Check sheet for the drawn part. Datum: minimum x, y, z corner. Units: mm. A direction names the side the tool comes from. Give positions to 0.01 mm unless a question says otherwise; leave off trailing zeros. Write each loop counter-clockwise with the first axis right and the second up, starting at its lowest first coordinate (ties: lowest second). Pieces come first, ordered by that corner, then holes.
(1) Thickness scan on line 1 along Z through (x, y) = (4, 1.35); line 2 along X through (y, z) = (5.5, 8.25); line 3 along X through (y, z) = (0.5, 4.5) (1 decimal). Record the ranges inside material, lowest first.
(2) Cross-section at D-D (z = 4). Record the boundary of the cut face in (x, y).
(3) Cross-section at B-B (y = 6.5). Record the boundary of the cut face in (x, z).
(4) Tool access check on the marked faces 5, 6 and 7. Record the directions out of +Z, -Z, +X, -X, +Y, -Y that give a thin tool (end or side, any length) a straight path to the whole face; none if there is none.
(5) Cross-section at C-C (y = 1.75). Record the boundary of the cut face in (x, z).
(6) Mould release check, pull along X, two halves, no side actions. Record for the marked faces 1, 2, 3 and 4: +X half, -X half, draft (parallel to the pull), parting line (faces both ways), or undercut.
(7) Depth check by flat-ended pin: P1, Ø1, axis at y = 6.5, z = 4.5, coming from the +X side; P2, Ø2.5, axis at x = 4, z = 4, coming from the -Y side; P3, Ø1.2, axis at x = 9, y = 5, coming from the -Z side; P4, Ø1.2, axis at x = 3, y = 1, coming from the +Z side. Enter the tip coordinate at first touch or a pass-through.
(8) Cross-section at A-A (x = 4). Record the boundary of the cut face in (y, z).
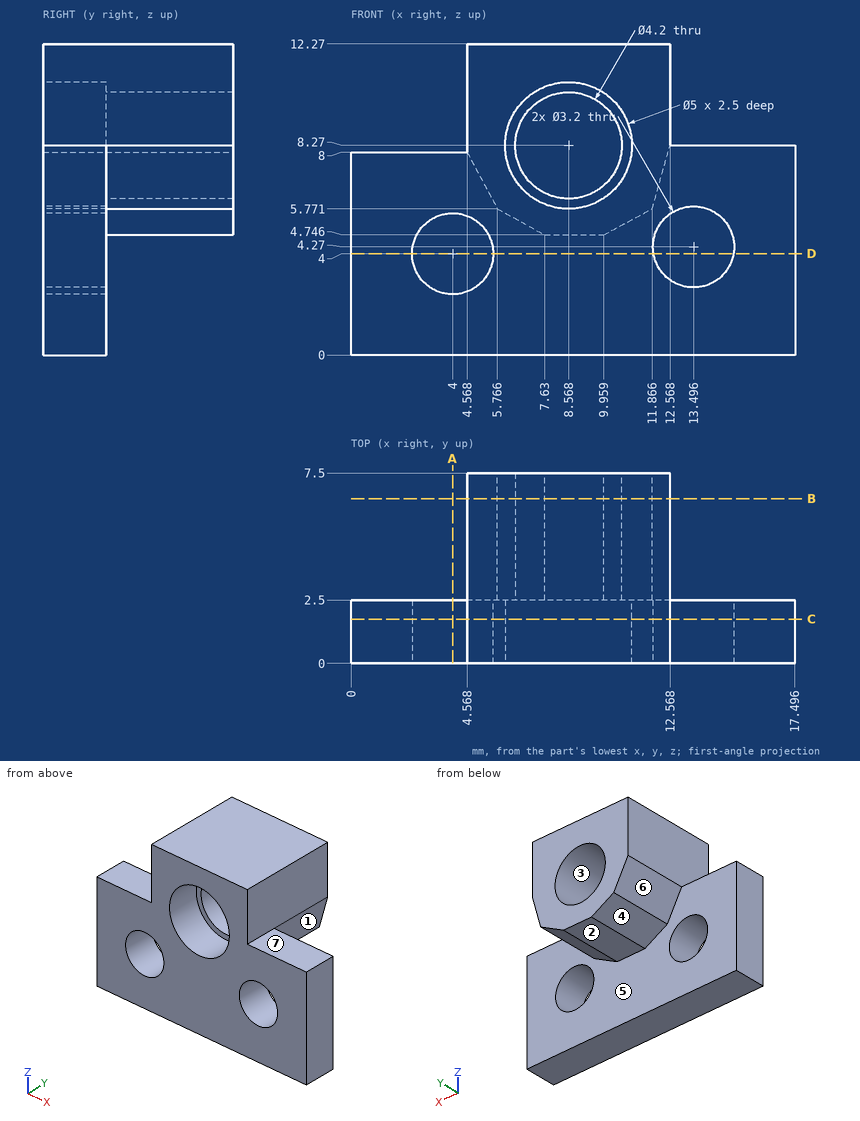
Reply:
1. line 1: z = 0 to 2.4, 5.6 to 8
1. line 2: x = 4.57 to 6.47, 10.67 to 12.56
1. line 3: x = 0 to 2.5, 5.5 to 11.9, 15.1 to 17.5
2. outline: (0, 0) - (2.4, 0) - (2.4, 2.5) - (0, 2.5) - close; (5.6, 0) - (11.92, 0) - (11.92, 2.5) - (5.6, 2.5) - close; (15.07, 0) - (17.5, 0) - (17.5, 2.5) - (15.07, 2.5) - close
3. outline: (4.57, 8) - (5.77, 5.77) - (7.63, 4.75) - (9.96, 4.75) - (11.87, 5.77) - (12.57, 8.27) - (12.57, 12.27) - (4.57, 12.27) - close; hole circle Ø4.2 at (8.57, 8.27)
4. face 5: -Z, +Y
4. face 6: -Z, -X, +Y
4. face 7: +Z, +X, +Y, -Y
5. outline: (0, 0) - (17.5, 0) - (17.5, 8.27) - (12.57, 8.27) - (12.57, 12.27) - (4.57, 12.27) - (4.57, 8) - (0, 8) - close; hole circle Ø3.2 at (4, 4); hole circle Ø5 at (8.57, 8.27); hole circle Ø3.2 at (13.5, 4.27)
6. face 1: +X half
6. face 2: draft
6. face 3: undercut
6. face 4: -X half
7. P1: stops at x = 10.43
7. P2: passes through
7. P3: stops at z = 4.75
7. P4: stops at z = 8
8. outline: (0, 0) - (2.5, 0) - (2.5, 2.4) - (0, 2.4) - close; (0, 5.6) - (2.5, 5.6) - (2.5, 8) - (0, 8) - close
